Can you work these out from the model? Positions are in its coordinate system, mm. A direction names the side the tool comes from. Give positions to 0.01 mm unless a question says otherwise; leave off trailing zeros. Loops run counter-clockwise (first coordinate to the right, second up) from the corner with the lowest first, then second, coordinate; pieces in that order, holes last. Notation, with made-up numbers: (-13, 53.25) -> (-9, 53.25) arc R17 ccw to (-9, 76.25) -> close; hole circle Ø10 at (0, 0). An arc over 180 degrees is marked (long way). Return JSON: item names as keys, results as strings. Group by question number.
Q1. Which directions (+Z, -Z, +X, -X, +Y, -Y) give clear straight access to the entire face, cutting with the end or side of a thin tool? Please do faces 4 (the cylindrical face through (-14.88, -10.74, 6.3)), 5 (the flat face through (35, 0, 5)), 6 (the flat face through (1, 0, -2)), 7 (the flat face through (-30, 0, 7)).
Q2. Suppose I cut it at B-B, the plane y = -7. Please give me the cut outline in (x, z).
Q3. Will these pins go through, and if not, where does the flat tip stop? pin 1 (3 mm diameter, centred on x = 35, y = 7, fed in from +Z); pin 2 (5 mm diameter, centred on x = -35.5, y = -4, fed in from +Z); pin 3 (2.5 mm diameter, centred on x = -26.46, y = -10.46, fed in from +Z); pin 4 (5.5 mm diameter, centred on y = 1.5, z = 8, fed in from -X).
Q4. I need wall thicknesses on line 1 along Y through (x, z) = (-26.5, 6); line 2 along X through (y, z) = (7, -0.9); line 3 along X through (y, z) = (3.75, 4). Which ranges of each line are inside material? Lowest first, please. Write a range as [from, to].
Q5. Suppose I cut it at C-C, the plane z = 3.25. Count the separate pieces of the cut face and the enclosed holes in it, and give its area (3 significant figures).
Q6. Suppose I cut it at A-A, the plane x = -35. Please give me the cut outline in (y, z), and give its area (3 significant figures).
Q7. Thinking about a two-plate mould opening in Y: for faces 1 (the flat face through (40, 0, 1)), 2 (the flat face through (26, -10, 0)), 3 (the flat face through (-1, -14, 4)), which applies, pulls with the +Y half, pulls with the -Y half, needs draft (parallel to the pull), parting line crosses it, or undercut?
Q8. Suppose I cut it at D-D, the plane y = 0. Please give me the cut outline in (x, z), and give its area (4 significant figures).
```python
from build123d import *

# Parameters (mm, degrees)
SKETCH1_W           = 60
SKETCH1_H           = 28
SKETCH1_R           = 4.1
SKETCH1_R_2         = 1.6
BOSS_EXTRUDE1_DEPTH = 10
SKETCH2_R           = 11
CUT_EXTRUDE1_DEPTH  = 7.5
SKETCH3_R           = 1.6
BOSS_EXTRUDE2_DEPTH = 2
SKETCH4_W           = 10
SKETCH4_H           = 28
SKETCH4_R           = 1.6
BOSS_EXTRUDE3_DEPTH = 5


with BuildPart() as part:
    # Sketch1 → Boss-Extrude1 (new body)
    with BuildSketch(Plane.XY):
        Rectangle(SKETCH1_W, SKETCH1_H)
        with Locations((12.5, 0)):
            Circle(SKETCH1_R, mode=Mode.SUBTRACT)
        with Locations((-12.5, 0)):
            Circle(SKETCH1_R, mode=Mode.SUBTRACT)
        with Locations((-26.464466094, 10.464466094)):
            Circle(SKETCH1_R_2, mode=Mode.SUBTRACT)
        with Locations((-26.464466094, -10.464466094)):
            Circle(SKETCH1_R_2, mode=Mode.SUBTRACT)
        with Locations((26.464466094, -10.464466094)):
            Circle(SKETCH1_R_2, mode=Mode.SUBTRACT)
        with Locations((26.464466094, 10.464466094)):
            Circle(SKETCH1_R_2, mode=Mode.SUBTRACT)
    extrude(amount=BOSS_EXTRUDE1_DEPTH)

    # Sketch2 → Cut-Extrude1 (cut)
    with BuildSketch(Plane.XY.offset(10)):
        with Locations((-12.5, 0)):
            Circle(SKETCH2_R)
    extrude(amount=-CUT_EXTRUDE1_DEPTH, mode=Mode.SUBTRACT)

    # Sketch3 → Boss-Extrude2 (add)
    with BuildSketch(Plane(origin=(0, 0, 0), x_dir=(-1, 0, 0), z_dir=(0, 0, -1))):
        Polygon((-30, 14), (-40, 14), (-40, -14), (-30, -14), (30, -14), (40, -14), (40, 14), (30, 14), align=None)
        with Locations((-35, 7)):
            Circle(SKETCH3_R, mode=Mode.SUBTRACT)
        with Locations((-35, -7)):
            Circle(SKETCH3_R, mode=Mode.SUBTRACT)
        with Locations((35, -7)):
            Circle(SKETCH3_R, mode=Mode.SUBTRACT)
        with Locations((35, 7)):
            Circle(SKETCH3_R, mode=Mode.SUBTRACT)
    extrude(amount=BOSS_EXTRUDE2_DEPTH)

    # Sketch4 → Boss-Extrude3 (add)
    with BuildSketch(Plane.XY):
        with Locations((35, 0)):
            Rectangle(SKETCH4_W, SKETCH4_H)
        with Locations((35, -7)):
            Circle(SKETCH4_R, mode=Mode.SUBTRACT)
        with Locations((35, 7)):
            Circle(SKETCH4_R, mode=Mode.SUBTRACT)
        with Locations((-35, 0)):
            Rectangle(SKETCH4_W, SKETCH4_H)
        with Locations((-35, -7)):
            Circle(SKETCH4_R, mode=Mode.SUBTRACT)
        with Locations((-35, 7)):
            Circle(SKETCH4_R, mode=Mode.SUBTRACT)
    extrude(amount=BOSS_EXTRUDE3_DEPTH)


solid = part.part
```
Ans:
{
 "1": {"face 4": "+Z", "face 5": "+Z, +X, +Y, -Y", "face 6": "-Z, +X, -X, +Y, -Y", "face 7": "+Z, -X, +Y, -Y"},
 "2": {"outline": "(-40, -2) -> (-36.6, -2) -> (-36.6, 5) -> (-40, 5) -> close; (-33.4, -2) -> (33.4, -2) -> (33.4, 5) -> (30, 5) -> (30, 10) -> (-4.01, 10) -> (-4.01, 2.5) -> (-20.99, 2.5) -> (-20.99, 10) -> (-30, 10) -> (-30, 5) -> (-33.4, 5) -> close; (36.6, -2) -> (40, -2) -> (40, 5) -> (36.6, 5) -> close"},
 "3": {"pin 1": "passes through", "pin 2": "stops at z = 5", "pin 3": "stops at z = 0", "pin 4": "stops at x = -30"},
 "4": {"line 1": "y = [-14, -12.06], [-8.86, 8.86], [12.06, 14]", "line 2": "x = [-40, -36.6], [-33.4, 33.4], [36.6, 40]", "line 3": "x = [-40, -22.84], [-2.16, 10.84], [14.16, 40]"},
 "5": {"separate pieces": "1", "enclosed holes": "10", "area": "1,740 mm^2"},
 "6": {"outline": "(-14, -2) -> (-8.6, -2) -> (-8.6, 5) -> (-14, 5) -> close; (-5.4, -2) -> (5.4, -2) -> (5.4, 5) -> (-5.4, 5) -> close; (8.6, -2) -> (14, -2) -> (14, 5) -> (8.6, 5) -> close", "area": "151 mm^2"},
 "7": {"face 1": "needs draft", "face 2": "undercut", "face 3": "pulls with the -Y half"},
 "8": {"outline": "(-40, -2) -> (40, -2) -> (40, 5) -> (30, 5) -> (30, 10) -> (16.6, 10) -> (16.6, 0) -> (8.4, 0) -> (8.4, 10) -> (-1.5, 10) -> (-1.5, 2.5) -> (-8.4, 2.5) -> (-8.4, 0) -> (-16.6, 0) -> (-16.6, 2.5) -> (-23.5, 2.5) -> (-23.5, 10) -> (-30, 10) -> (-30, 5) -> (-40, 5) -> close", "area": "592.5 mm^2"}
}
